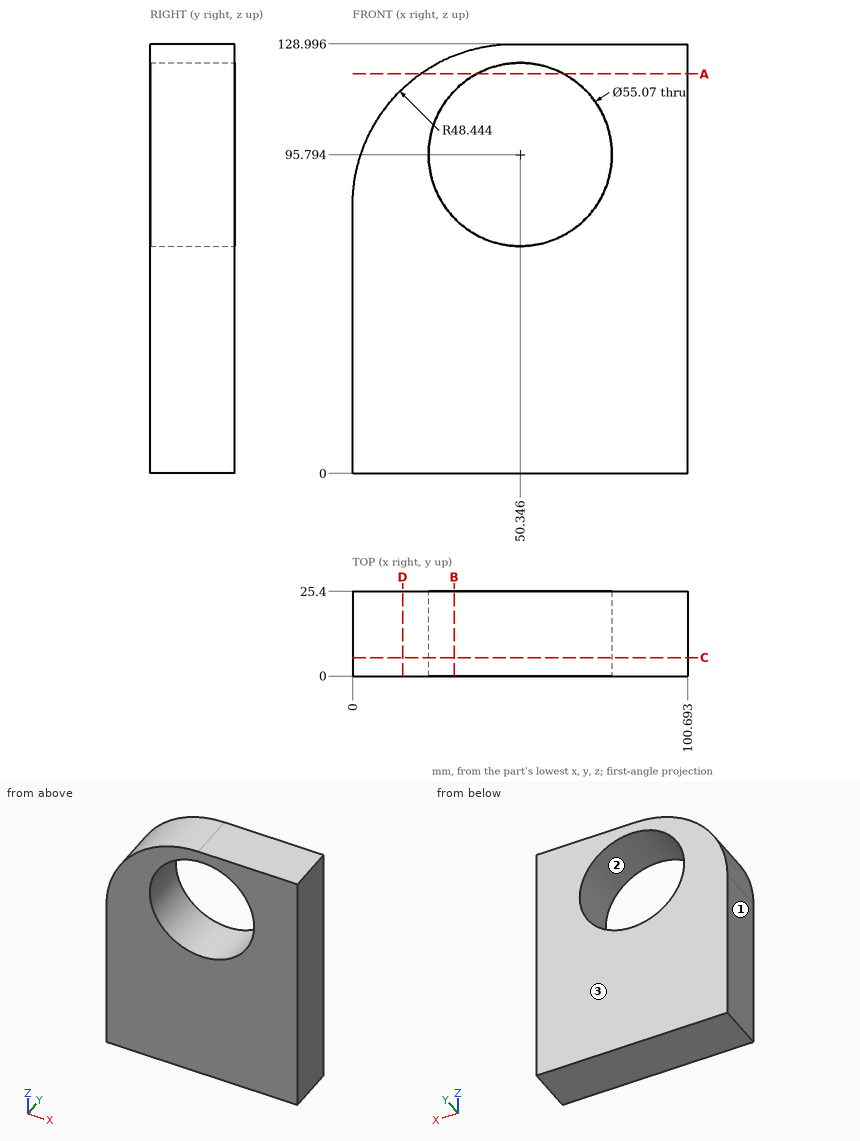
Answer from the drawing. Dimensions are ordinates in mm from the lowest x, y and z of the part. Round coordinates to 2 decimals unless told otherwise and drop trailing zeros. Loops run counter-clockwise (first coordinate to the right, second up) from the corner with the lowest first, then second, coordinate; pieces in that order, holes last.
1) A cutting plane is placed at D-D on x = 15. Determine the outline of the cut face in (y, z).
Outcome:
outline: (0, 0) - (25.4, 0) - (25.4, 115.6) - (0, 115.6) - close
2) A cutting plane is placed at A-A on z = 120. Determine the outline of the cut face in (x, y) (1 decimal), plus the area to 3 significant figures.
Outcome:
outline: (20.3, 0) - (37.2, 0) - (37.2, 25.4) - (20.3, 25.4) - close; (63.5, 0) - (100.7, 0) - (100.7, 25.4) - (63.5, 25.4) - close
area: 1,370 mm2
3) For a pull along X with two mould halves and no side action, classify the marked faces 1, 2 and 3 as released by +X, released by -X, zero draft, split by the parting line, or undercut.
Outcome:
face 1: released by -X
face 2: undercut
face 3: zero draft
4) A cutting plane is placed at C-C on y = 5.5. Determine the outline of the cut face in (x, z) (1 decimal), plus the area to 3 significant figures.
Outcome:
outline: (0, 0) - (100.7, 0) - (100.7, 129) - (48.4, 129) arc R48.4 ccw to (0, 80.6) - close; hole circle Ø55.1 at (50.3, 95.8)
area: 10,100 mm2
5) A cutting plane is placed at B-B on x = 30.5. Determine the outline of the cut face in (y, z).
Outcome:
outline: (0, 0) - (25.4, 0) - (25.4, 76.71) - (0, 76.71) - close; (0, 114.88) - (25.4, 114.88) - (25.4, 125.55) - (0, 125.55) - close
6) Given P1, Ø4, axis at y = 17, z = 86.5, coming from the -X side; P2, Ø8, axis at y = 6.5, z = 98.5, coming from the -X side, each flat-ended and moving along its own axis, determine where each tip first touches the part or whether it passes through.
Outcome:
P1: stops at x = 0.16
P2: stops at x = 2.05
7) Consider line 1 (Z direction, x = 51, y = 15.25) (1 decimal); line 2 (Z direction, x = 37, y = 20.75) (1 decimal); line 3 (Z direction, x = 19.5, y = 3.5). Determine where each line is inside the solid, lowest interval first.
Outcome:
line 1: z = 0 to 68.3, 123.3 to 129
line 2: z = 0 to 71.7, 119.9 to 127.6
line 3: z = 0 to 119.4
